Job drawing, mm, ordinate dimensions from the low corner. One solid piece. A direction names the side the tool comes from. Give positions to 0.01 mm unless a question says otherwise; leave off trailing zeros. Loops run counter-clockwise (first coordinate to the right, second up) from the corner with the lowest first, then second, coordinate; pieces in that order, holes last. Notation, with made-up numbers: (34, 38) - (68, 38) arc R36 ccw to (68, 75) - close; hole circle Ø4 at (-4, 4). An arc over 180 degrees is marked (long way). Answer as CSV lines item,"result". Start each with the question number.
Item 1: Saw through at D-D on x = 22.5. Give the cut face in (y, z).
Item 2: Saw through at B-B on x = 30. Give the cut face in (y, z), plus the area to 3 significant figures.
Item 3: Drill centre lines: L1, parallel to Z at x = 31, y = 15; L2, parallel to Y at x = 30, z = 4.5; L3, parallel to X at y = 10, z = 9.75. Where is each one in solid material? Low to high. Write a range as from..to.
Item 4: Pin check, flat tip, straight feed: pin 1 (4 mm diameter, centred on x = 23, z = 5.5, fed in from +Y). Stop position of the tip, or through.
Item 5: Pull direction Z, two halves, no side cores. Call the marked faces 1, 2 and 3: pulls with the +Z half, pulls with the -Z half, needs draft (parallel to the pull), parting line crosses it, or undercut.
Item 6: Tool access for the marked faces 4 and 5: list every direction of +Z, -Z, +X, -X, +Y, -Y with a clear straight run to the whole face (end or side of a thin tool).
Item 7: Saw through at A-A on y = 15.75. Give the cut face in (x, z).
Item 8: Saw through at C-C on z = 6.25. Give the cut face in (x, y).
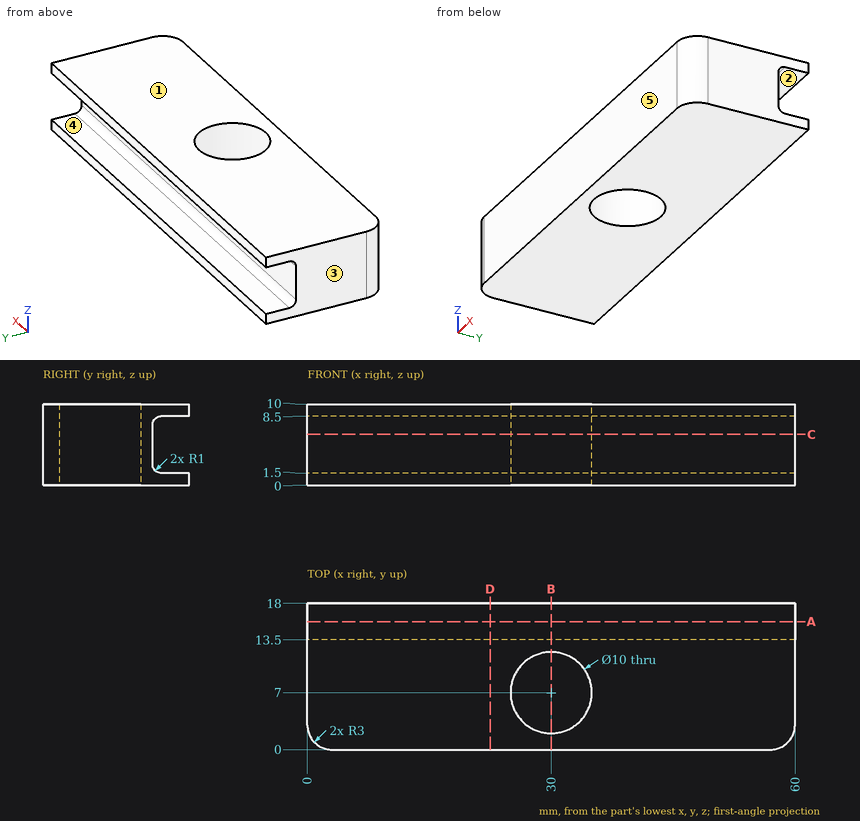
Responses:
1,outline,"(0, 0) - (18, 0) - (18, 1.5) - (14.5, 1.5) arc R1 cw to (13.5, 2.5) - (13.5, 7.5) arc R1 cw to (14.5, 8.5) - (18, 8.5) - (18, 10) - (0, 10) - close"
2,outline,"(0, 0) - (2, 0) - (2, 10) - (0, 10) - close; (12, 0) - (18, 0) - (18, 1.5) - (14.5, 1.5) arc R1 cw to (13.5, 2.5) - (13.5, 7.5) arc R1 cw to (14.5, 8.5) - (18, 8.5) - (18, 10) - (12, 10) - close"
2,area,"48.9 mm2"
3,L1,"0..1.5, 8.5..10"
3,L2,"0..2, 12..13.5"
3,L3,"0..26, 34..60"
4,pin 1,"y = 13.5"
5,face 1,"pulls with the +Z half"
5,face 2,"undercut"
5,face 3,"needs draft"
6,face 4,"+X, -X, +Y"
6,face 5,"+Z, -Z, +X, -X, -Y"
7,outline,"(0, 0) - (60, 0) - (60, 1.5) - (0, 1.5) - close; (0, 8.5) - (60, 8.5) - (60, 10) - (0, 10) - close"
8,outline,"(0, 3) arc R3 ccw to (3, 0) - (57, 0) arc R3 ccw to (60, 3) - (60, 13.5) - (0, 13.5) - close; hole circle Ø10 at (30, 7)"
